Autodesk Inventor part; units mm, degrees
ref_plane "YZ Plane" through (0, 0, 0) normal (1, 0, 0) x (0, 1, 0)
ref_plane "XZ Plane" through (0, 0, 0) normal (0, 1, 0) x (-1, 0, 0)
ref_plane "XY Plane" through (0, 0, 0) normal (0, 0, 1) x (1, 0, 0)
sketch "Sketch5" plane through (0, 0, 0) normal (0, 0, 1) x (1, 0, 0)
  line L0 (8.1925, 0) -> (8.1925, 2.0926)
  point P0 (0, 0)
sketch "Sketch6" plane through (0, 0, 0) normal (0, 0, 1) x (1, 0, 0)
  circle A0 centre (8.1925, 2.0909) radius 1.5875
  point P0 (0, 0)
  dimension "d2" = 3.175
sketch "Sketch7" plane through (0, 0, 0) normal (0, 0, 1) x (1, 0, 0)
  circle A0 centre (8.1923, 2.092) radius 1.5921
  circle A1 centre (8.1923, 2.092) radius 2.9715
  circle A2 centre (24.0624, -39.8776) radius 1.5875
  circle A3 centre (24.0624, -39.8776) radius 3.9111
  line L0 (6.4132, -0.2881) -> (21.2107, -37.2008)
  line L1 (26.9141, -37.2008) -> (10.9559, 3.184)
  point P0 (0, 0)
  dimension "d4" = 3.175
extrude "Extrusion1" add sketch "Sketch7" along normal blind 3.175
properties part number "LowerArm"
Here's how the part is built. I have some questions about the finished solid (model axes, mm). Coordinates: 2 decimals unless noted, no trailing zeros. Loops run counter-clockwise (first coordinate to the right, second up) from the corner with the lowest first, then second, coordinate; pieces in that order, holes last. Notation, with made-up numbers: (18, 70.25) - (72, 70.25) arc R29 ccw to (72, 102.25) - close; hole circle Ø6 at (71.25, 23.25). An arc over 180 degrees is marked (long way). Return JSON: item names as keys, results as strings. Group by question number.
Item 1: If we section it at B-B on z = 1.5: Write out the boundary of the cut face in (x, y) (1 decimal), and give its area (3 significant figures).
Item 2: If we section it at D-D on x = 16.5: Write out the boundary of the cut face in (y, z) (3 decimals).
Item 3: We'd pull the mould along X, two halves only. Please class faces 1 (the face through (13.71, -18.49, 1.57)), 2 (the face through (17, -19, 3.175)), 3 (the face through (9.71, 1.61, 1.57)): +X half, -X half, draft (parallel to the pull), parting line (faces both ways), or undercut.
Item 4: I need wall thicknesses on line 1 (X direction, y = -40, z = 1.85); line 2 (Y direction, x = 6.75, z = 1.2); line 3 (Y direction, x = 10.25, z = 2.2). Which ranges of each line are inside material? Lowest first, please. Write a range as from..to.
Item 5: Will this pin go through, and if not, where does the flat tip stop? P1, Ø1.5, axis at y = -9.5, z = 0.5, coming from the -X side.
Item 6: If we section it at A-A on x = 23.25: Write out the boundary of the cut face in (y, z) (3 decimals).
Item 7: If we section it at C-C on y = -12: Write out the boundary of the cut face in (x, z) (3 decimals).
Calculated:
{
 "1": {"outline": "(6.4, -0.3) - (21.2, -37.2) arc R3.9 ccw (long way) to (26.9, -37.2) - (11, 3.2) arc R3 ccw (long way) to start; hole circle Ø3.2 at (8.2, 2.1); hole circle Ø3.2 at (24.1, -39.9)", "area": "271 mm^2"},
 "2": {"outline": "(-25.45, 0) - (-10.846, 0) - (-10.846, 3.175) - (-25.45, 3.175) - close"},
 "3": {"face 1": "-X half", "face 2": "draft", "face 3": "undercut"},
 "4": {"line 1": "x = 20.15..22.48, 25.65..27.97", "line 2": "y = -1.13..1.42, 2.77..4.69", "line 3": "y = -9.86..4.24"},
 "5": {"P1": "stops at x = 9.81"},
 "6": {"outline": "(-43.703, 0) - (-41.241, 0) - (-41.241, 3.175) - (-43.703, 3.175) - close; (-38.514, 0) - (-27.928, 0) - (-27.928, 3.175) - (-38.514, 3.175) - close"},
 "7": {"outline": "(11.108, 0) - (16.956, 0) - (16.956, 3.175) - (11.108, 3.175) - close"}
}
